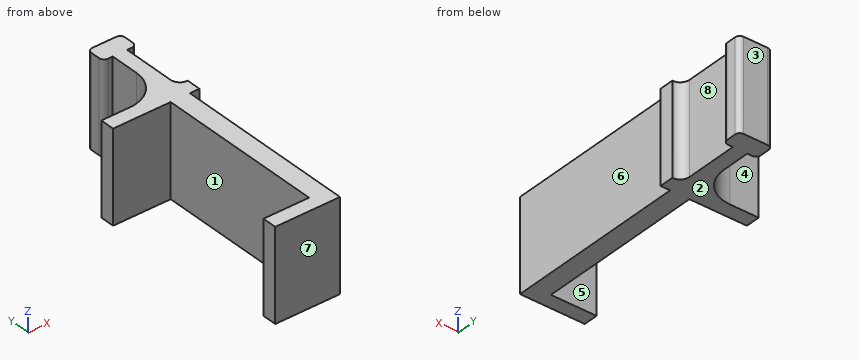
from build123d import *

# Parameters (mm, degrees)
PAD121_DEPTH   = 19
PAD121_FACE5_W = 4
PAD121_FACE5_H = 19
PAD127_DEPTH   = 0.3
SKETCH126_W    = 18
SKETCH126_H    = 19
PAD128_DEPTH   = 3
SKETCH127_W    = 3
SKETCH127_H    = 19
PAD129_DEPTH   = 15
SKETCH128_W    = 7
SKETCH128_H    = 4
PAD130_DEPTH   = 19
FILLET056_R    = 1
FILLET057_R    = 1.9
FILLET058_R    = 7


with BuildPart() as part:
    # Sketch119 → Pad121 (new body)
    with BuildSketch(Plane.XY):
        Polygon((0, 0), (-13.5, 0), (-13.5, 3), (-4, 3), (-4, 38), (0, 38), align=None)
    extrude(amount=PAD121_DEPTH)

    # Pad121 Face5 → Pad127 (add)
    with BuildSketch(Plane(origin=(-2, 38, 9.5), x_dir=(1, 0, 0), z_dir=(0, 1, 0))):
        Rectangle(PAD121_FACE5_W, PAD121_FACE5_H)
    extrude(amount=PAD127_DEPTH)

    # Sketch126 (on Face5 of Pad127) → Pad128 (join)
    with BuildSketch(Plane(origin=(0, 38.3, 0), x_dir=(-1, 0, 0), z_dir=(0, 1, 0))):
        with Locations((7, 9.5)):
            Rectangle(SKETCH126_W, SKETCH126_H)
    extrude(amount=PAD128_DEPTH)

    # Sketch127 (on Face3 of Pad128) → Pad129 (join)
    with BuildSketch(Plane(origin=(0, 41.3, 0), x_dir=(-1, 0, 0), z_dir=(0, 1, 0))):
        with Locations((1.5, 9.5)):
            Rectangle(SKETCH127_W, SKETCH127_H)
    extrude(amount=PAD129_DEPTH)

    # Sketch128 (on Face15 of Pad129) → Pad130 (join)
    with BuildSketch(Plane(origin=(0, 0, 0), x_dir=(1, 0, 0), z_dir=(0, 0, -1))):
        with Locations((-1.5, -56.3)):
            Rectangle(SKETCH128_W, SKETCH128_H)
    extrude(amount=-PAD130_DEPTH)

    # Fillet056
    fillet056_edges = [part.edges().sort_by_distance(p)[0] for p in [
        (2, 58.3, 9.5),
        (2, 54.3, 9.5),
        (-5, 58.3, 9.5),
        (-5, 54.3, 9.5),
    ]]
    fillet(fillet056_edges, radius=FILLET056_R)

    # Fillet057
    fillet057_edges = [part.edges().sort_by_distance(p)[0] for p in [
        (0, 41.3, 9.5),
    ]]
    fillet(fillet057_edges, radius=FILLET057_R)

    # Fillet058
    fillet058_edges = [part.edges().sort_by_distance(p)[0] for p in [
        (-3, 41.3, 9.5),
    ]]
    fillet(fillet058_edges, radius=FILLET058_R)


solid = part.part
The model under review builds one solid part; all positions refer to its coordinate system, in mm. Face numbers are marked on the shaded views. A direction names the side the tool comes from. Give positions to 0.01 mm unless a question says otherwise; leave off trailing zeros. Order: outer loops, then holes, each group sorted by start corner. A loop starts at its lowest first (then second) coordinate and runs counter-clockwise, first axis right, second up. Notation, with made-up numbers: (58.5, -35.5) -> (112.5, -35.5) arc R18 ccw to (112.5, -20.5) -> close; hole circle Ø5 at (67.25, 82.25). An arc over 180 degrees is marked (long way). Write item = value, one per line. Start each with the question number.
(1) Tool access review of the marked faces 4, 5, 6, 7 and 8: name each direction out of +Z, -Z, +X, -X, +Y, -Y from which nothing blocks a thin tool from reaching the whole face with its end or side.
(2) Take a section at B-B (z = 3). Write out the cut boundary in (x, y), plus the area to 3 significant figures.
(3) For L1, parallel to Y at x = -13, z = 10.5; L2, parallel to X at y = 14, z = 4.25; L3, parallel to Y at x = -8.5, z = 5.75, list the stretches that pass through material, from the lowest coordinate up. Write a range as from..to.
(4) Draft analysis for pull direction Y (two halves, no side actions). For the marked faces 1, 2 and 3, state which applies: +Y half, -Y half, draft (parallel to the pull), parting line (faces both ways), or undercut.
(5) Take a section at C-C (x = -5.75). Write out the cut boundary in (y, z).
(6) Take a section at D-D (y = 51.5). Write out the cut boundary in (x, z).
(7) Take a section at A-A (x = -12). Write out the cut boundary in (y, z), plus the area to 3 significant figures.
(8) For pin 1 Ø2.5 at (y, z) = (1, 14) entering from -X; pin 2 Ø5 at (x, z) = (-12.5, 8) entering from +Y; pin 3 Ø10 at (x, z) = (-11.5, 13) entering from +Y, all flat-tipped, find the tip position at first contact; note any pin that passes through.
Returned:
q1.face_4 = +Z, -Z, -X, +Y
q1.face_5 = +Z, -Z, -X
q1.face_6 = +Z, -Z, +X, -Y
q1.face_7 = +Z, -Z, +X, -X, -Y
q1.face_8 = +Z, -Z, +X
q2.outline = (-16, 38.3) -> (-4, 38.3) -> (-4, 3) -> (-13.5, 3) -> (-13.5, 0) -> (0, 0) -> (0, 38.3) -> (2, 38.3) -> (2, 41.3) -> (1.9, 41.3) arc R1.9 cw to (0, 43.2) -> (0, 54.3) -> (1, 54.3) arc R1 ccw to (2, 55.3) -> (2, 57.3) arc R1 ccw to (1, 58.3) -> (-4, 58.3) arc R1 ccw to (-5, 57.3) -> (-5, 55.3) arc R1 ccw to (-4, 54.3) -> (-3, 54.3) -> (-3, 48.3) arc R7 cw to (-10, 41.3) -> (-16, 41.3) -> close
q2.area = 313 mm²
q3.L1 = 0..3, 38.3..41.3
q3.L2 = -4..0
q3.L3 = 0..3, 38.3..41.46
q4.face_1 = undercut
q4.face_2 = draft
q4.face_3 = +Y half
q5.outline = (0, 0) -> (3, 0) -> (3, 19) -> (0, 19) -> close; (38.3, 0) -> (42.74, 0) -> (42.74, 19) -> (38.3, 19) -> close
q6.outline = (-3, 0) -> (0, 0) -> (0, 19) -> (-3, 19) -> close
q7.outline = (0, 0) -> (3, 0) -> (3, 19) -> (0, 19) -> close; (38.3, 0) -> (41.3, 0) -> (41.3, 19) -> (38.3, 19) -> close
q7.area = 114 mm²
q8.pin_1 = -13.5
q8.pin_2 = 41.3
q8.pin_3 = 42.24
